Print and shaded views of the part. All mm, measured from the part's lowest x, y and z. A direction names the side the tool comes from. Give positions to 0.01 mm unless a question says otherwise; leave off trailing zeros. Write each loop counter-clockwise with the first axis right and the second up, starting at its lowest first coordinate (ties: lowest second). Pieces come first, ordered by that corner, then holes. Notation, with made-up numbers: M 25,-1 L 66,-1 A36 cw 66,36 Z; hole C 35,58 d1. An arc over 180 degrees is marked long. One line per question, with ' | ' between items. Start each with the question number.
1. Cut at A-A, the plane y = 18. Write the cut outline in (x, z), then the cut area to 3 significant figures.
2. Pull direction Z, two halves, no side cores. Call the marked faces 3, 4 and 5: released by +Z, released by -Z, zero draft, split by the parting line, or undercut.
3. Cut at B-B, the plane z = 21. Write the cut outline in (x, y).
4. Cut at D-D, the plane y = 30. Write the cut outline in (x, z), then the cut area to 3 significant figures.
5. Wall check: L1, parallel to X at y = 42, z = 11; L2, parallel to Z at x = 6.5, y = 26.5; L3, parallel to Y at x = 17.5, z = 30.5. Give the ranges that are in metal, low to high.
6. Cut at C-C, the plane x = 2. Write the cut outline in (y, z).
7. Which spindle directions (+Z, -Z, +X, -X, +Y, -Y) get a long thin tool onto all of the face, cutting with end or side? Do the marked faces 1 and 2. Say none if no direction does.
8. Flat gauge pin, fed straight in: pin 1 (5 mm diameter, centred on x = 15, z = 11, fed in from -Y). Where does the tip first touch, or does it go through?
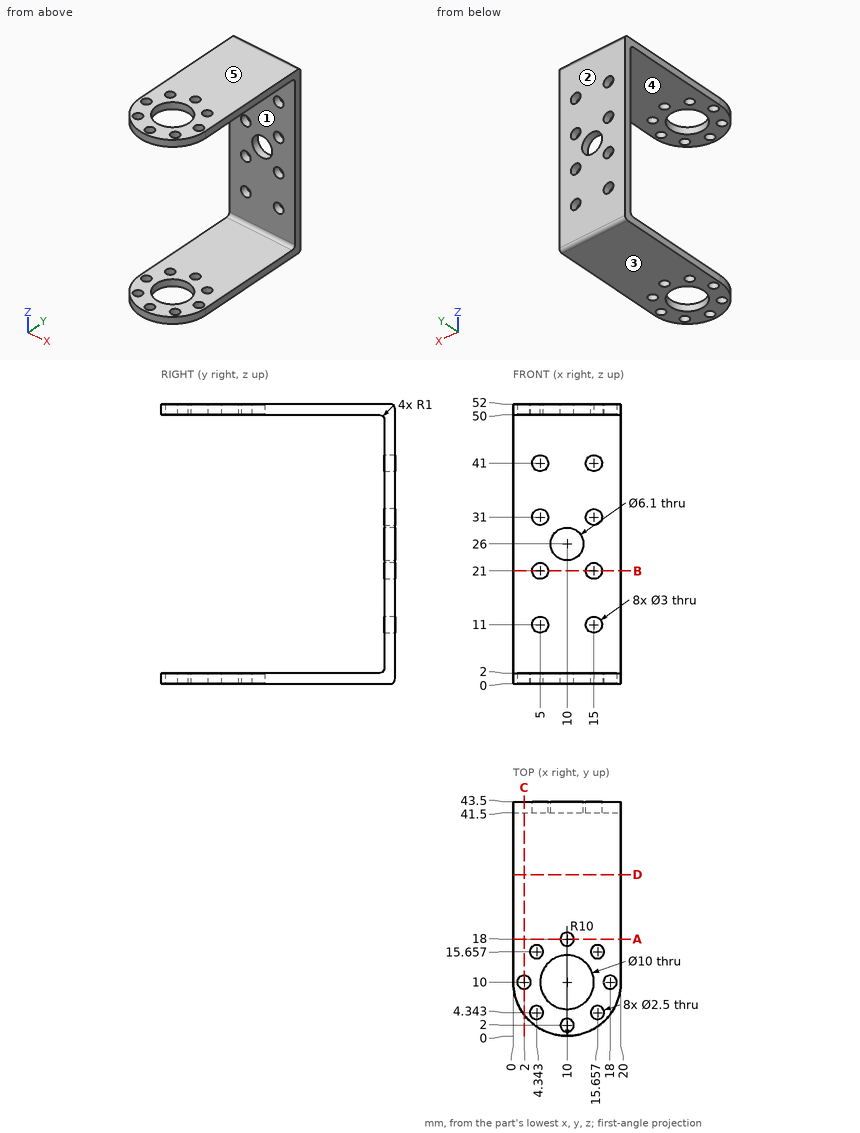
Here are the results:
1) outline: M 0,0 L 8.75,0 L 8.75,2 L 0,2 Z; M 0,50 L 8.75,50 L 8.75,52 L 0,52 Z; M 11.25,0 L 20,0 L 20,2 L 11.25,2 Z; M 11.25,50 L 20,50 L 20,52 L 11.25,52 Z | area: 70.0 mm^2
2) face 3: released by -Z | face 4: undercut | face 5: released by +Z
3) outline: M 0,41.5 L 3.5,41.5 L 3.5,43.5 L 0,43.5 Z; M 6.5,41.5 L 13.5,41.5 L 13.5,43.5 L 6.5,43.5 Z; M 16.5,41.5 L 20,41.5 L 20,43.5 L 16.5,43.5 Z
4) outline: M 0,0 L 20,0 L 20,2 L 0,2 Z; M 0,50 L 20,50 L 20,52 L 0,52 Z | area: 80.0 mm^2
5) L1: 0 to 3.5, 6.5 to 13.5, 16.5 to 20 | L2: 0 to 2, 50 to 52 | L3: 41.5 to 43.5
6) outline: M 4,0 L 8.75,0 L 8.75,2 L 4,2 Z; M 4,50 L 8.75,50 L 8.75,52 L 4,52 Z; M 11.25,0 L 42.5,0 A1 ccw 43.5,1 L 43.5,51 A1 ccw 42.5,52 L 11.25,52 L 11.25,50 L 40.5,50 A1 cw 41.5,49 L 41.5,3 A1 cw 40.5,2 L 11.25,2 Z
7) face 1: +X, -X, -Y | face 2: +Z, -Z, +X, -X, +Y
8) pin 1: y = 41.5
